```python
from build123d import *

# Parameters (mm, degrees)
F0_W     = 717.55
F0_H     = 539.75
F1_DEPTH = 12.7
F2_SIZE  = 50.8
F4_D     = 76.2


with BuildPart() as f1:
    # F0 (on Top) → F1 (new body)
    with BuildSketch(Plane.XY):
        with Locations((91.337793, 114.312262)):
            Rectangle(F0_W, F0_H)
    extrude(amount=F1_DEPTH)

    # F2
    f2_edges = [f1.edges().sort_by_distance(p)[0] for p in [
        (450.112793, 384.187262, 6.35),
        (450.112793, -155.562738, 6.35),
        (-267.437207, -155.562738, 6.35),
        (-267.437207, 384.187262, 6.35),
    ]]
    chamfer(f2_edges, length=F2_SIZE)

    # F4 (through all)
    with Locations(Plane(origin=(0, 0, 0), x_dir=(1, 0, 0), z_dir=(0, 0, -1))):
        with Locations((91.337793, -114.312262)):
            Hole(F4_D / 2)


solid = f1.part
```
Check sheet for the modelled part. Datum: model origin and axes. Units: mm. Give positions to 0.01 mm unless a question says otherwise; leave off trailing zeros. Loops run counter-clockwise (first coordinate to the right, second up) from the corner with the lowest first, then second, coordinate; pieces in that order, holes last. Notation, with made-up numbers: M 28,13.25 L 43,13.25 A22 ccw 43,32.25 Z; hole C 48,16.25 d10. An arc over 180 degrees is marked long. Answer in a Markdown table with one row per item.
1) Cross-section at A-A (z = 5). Enter the section's corners in (x, y), plus the area to 3 significant figures.
Solutions:
| item | result |
|---|---|
| outline | M -267.44,-104.76 L -216.64,-155.56 L 399.31,-155.56 L 450.11,-104.76 L 450.11,333.39 L 399.31,384.19 L -216.64,384.19 L -267.44,333.39 Z; hole C 91.34,114.31 d76.2 |
| area | 378,000 mm^2 |
2) Mould release check, pull along Y, two halves, no side actions. Record for faces 1 (the face through (424.4, 359.1, 6.3)), 2 (the face through (129.4, 112.6, 6.4)), 3 (the face through (-241.7, -130.5, 6.3)): released by +Y, released by -Y, zero draft, split by the parting line, or undercut.
Solutions:
| item | result |
|---|---|
| face 1 | released by +Y |
| face 2 | undercut |
| face 3 | released by -Y |
3) Thickness scan on line 1 (X direction, y = 85, z = 3.25); line 2 (X direction, y = 136, z = 2); line 3 (X direction, y = -116, z = 9.75). Record the ranges inside material, lowest first.
Solutions:
| item | result |
|---|---|
| line 1 | x = -267.44 to 67, 115.68 to 450.11 |
| line 2 | x = -267.44 to 60.01, 122.66 to 450.11 |
| line 3 | x = -256.2 to 438.88 |
4) Cross-section at B-B (y = 86.5). Enter the section's corners in (x, z).
Solutions:
| item | result |
|---|---|
| outline | M -267.44,0 L 65.3,0 L 65.3,12.7 L -267.44,12.7 Z; M 117.38,0 L 450.11,0 L 450.11,12.7 L 117.38,12.7 Z |
